Design review of the part built by this model. Coordinates are the model's own, in mm. A direction names the side the tool comes from. Coordinates: 2 decimals unless noted, no trailing zeros. Write each loop counter-clockwise with the first axis right and the second up, starting at its lowest first coordinate (ties: lowest second). Pieces come first, ordered by that corner, then holes.
Q1. Take a section at A-A, the plane x = 11.8. Write out the cut boundary in (y, z), plus the area to 3 significant figures.
Q2. Take a section at B-B, the plane y = 3.5. Write out the cut boundary in (x, z), plus the area to 3 significant figures.
Q3. For pin 1 Ø11 at (x, y) = (-5.5, -1.5) entering from +Z; pin 2 Ø2 at (y, z) = (10.5, -39) entering from +X; pin 3 Ø5 at (x, y) = (-3, 11.5) entering from +Z, all flat-tipped, find the tip position at first contact; note any pin that passes through.
Q4. Take a section at D-D, the plane z = -24. Write out the cut boundary in (x, y).
Q5. For L1, parallel to X at y = 0.25, z = -9.45; L2, parallel to X at y = 5.25, z = 35 (3 decimals); L3, parallel to X at y = 12.25, z = 33.5, list the stretches that pass through material, from the lowest coordinate up.
Q6. For faces 4 (the cylindrical face through (13.11, 0.07, -8.62)), 5 (the flat face through (16.3, 10, 13)), list the 3-axis set-ups (+Z, -Z, +X, -X, +Y, -Y) from which the entire face can be reached by the end or side of a thin tool; tool diameter is ignored.
Q7. Take a section at C-C, the plane z = -9.45. Write out the cut boundary in (x, y).
Q8. The part is to be moulded in two halves that separate along Z. For faces 1 (the flat face through (-17, 10, -38)), 2 (the flat face through (0, 0, 40)), 3 (the flat face through (30, 5, 0)), say which applies: released by +Z, released by -Z, zero draft, split by the parting line, or undercut.
from build123d import *

# Parameters (mm, degrees)
SKETCH1_W           = 60
SKETCH1_H           = 80
BOSS_EXTRUDE1_DEPTH = 5
FILLET1_R           = 10
SKETCH3_R           = 1.55
CUT_EXTRUDE11_DEPTH = 10
BOSS_EXTRUDE2_DEPTH = 10
BOSS_EXTRUDE3_DEPTH = 10


with BuildPart() as part:
    # Sketch1 → Boss-Extrude1 (new, symmetric)
    with BuildSketch(Plane(origin=(0, 0, 0), x_dir=(1, 0, 0), z_dir=(0, 1, 0))):
        Rectangle(SKETCH1_W, SKETCH1_H)
    extrude(amount=BOSS_EXTRUDE1_DEPTH, both=True)

    # Fillet1
    fillet1_edges = [part.edges().sort_by_distance(p)[0] for p in [
        (-30, 0, -40),
        (30, 0, -40),
        (30, 0, 40),
        (-30, 0, 40),
    ]]
    fillet(fillet1_edges, radius=FILLET1_R)

    # Sketch3 → Cut-Extrude11 (cut)
    with BuildSketch(Plane(origin=(0, 5, 0), x_dir=(1, 0, 0), z_dir=(0, 1, 0))):
        with Locations(Location((-11.8, 9.45, 0), (0, 0, 270))):
            Circle(SKETCH3_R)
        with Locations(Location((11.8, 9.45, 0), (0, 0, 270))):
            Circle(SKETCH3_R)
        with Locations(Location((-11.8, -37.55, 0), (0, 0, 270))):
            Circle(SKETCH3_R)
        with Locations(Location((11.8, -37.55, 0), (0, 0, 270))):
            Circle(SKETCH3_R)
    extrude(amount=-CUT_EXTRUDE11_DEPTH, mode=Mode.SUBTRACT)

    # Sketch6 → Boss-Extrude2 (add)
    with BuildSketch(Plane(origin=(0, 5, 0), x_dir=(1, 0, 0), z_dir=(0, 1, 0))):
        with BuildLine():
            Line((30, -30), (30, 30))
            ThreePointArc((30, 30), (27.071067812, 37.071067812), (20, 40))
            Line((20, 40), (14.5, 40))
            Line((14.5, 40), (14.5, 38))
            Line((14.5, 38), (20, 38))
            ThreePointArc((20, 38), (25.656854249, 35.656854249), (28, 30))
            Line((28, 30), (28, -30))
            ThreePointArc((28, -30), (25.652656249, -35.661049137), (19.988130666, -37.999991195))
            Line((19.988130666, -37.999991195), (14.301118682, -38.071478623))
            Line((14.301118682, -38.071478623), (14.285233791, -38.789415009))
            Line((14.285233791, -38.789415009), (12.98648686, -40.088161941))
            Line((12.98648686, -40.088161941), (20, -40))
            ThreePointArc((20, -40), (27.071067812, -37.071067812), (30, -30))
        make_face()
        with BuildLine():
            Line((-30, 30), (-30, -30))
            ThreePointArc((-30, -30), (-27.071067812, -37.071067812), (-20, -40))
            Line((-20, -40), (-13.014230023, -40.088161941))
            Line((-13.014230023, -40.088161941), (-14.314872692, -38.748440589))
            Line((-14.314872692, -38.748440589), (-14.314872692, -38.071588283))
            Line((-14.314872692, -38.071588283), (-19.988083532, -37.999991125))
            ThreePointArc((-19.988083532, -37.999991125), (-25.652639572, -35.661065789), (-28, -30))
            Line((-28, -30), (-28, 30))
            ThreePointArc((-28, 30), (-25.656854249, 35.656854249), (-20, 38))
            Line((-20, 38), (-14.5, 38))
            Line((-14.5, 38), (-14.5, 40))
            Line((-14.5, 40), (-20, 40))
            ThreePointArc((-20, 40), (-27.071067812, 37.071067812), (-30, 30))
        make_face()
    extrude(amount=BOSS_EXTRUDE2_DEPTH)

    # Sketch5 → Boss-Extrude3 (add)
    with BuildSketch(Plane(origin=(0, 5, 0), x_dir=(1, 0, 0), z_dir=(0, 1, 0))):
        Polygon((14.285233791, -38.789415009), (14.3, 10.507634941), (12.98648686, 11.821148081), (-13.014230023, 11.821148081), (-14.31369616, 10.516205754), (-14.314872692, 10.512459037), (-14.314872692, -38.748440589), (-16.314872692, -38.748440589), (-16.314872692, 10.819094366), (-15.842590188, 11.515908447), (-13.84512164, 13.821148081), (13.814913984, 13.821148081), (16.300248159, 11.335813907), (16.300248159, -38.789415009), align=None)
    extrude(amount=BOSS_EXTRUDE3_DEPTH)


solid = part.part
Responses:
1. outline: (-5, -40) - (5, -40) - (5, -13.82) - (15, -13.82) - (15, -11.82) - (5, -11.82) - (5, -11) - (-5, -11) - close; (-5, -7.9) - (5, -7.9) - (5, 36) - (-5, 36) - close; (-5, 39.1) - (5, 39.1) - (5, 40) - (-5, 40) - close
1. area: 758 mm2
2. outline: (-30, -30) arc R10 ccw to (-20, -40) - (20, -40) arc R10 ccw to (30, -30) - (30, 30) arc R10 ccw to (20, 40) - (-20, 40) arc R10 ccw to (-30, 30) - close; hole circle Ø3.1 at (-11.8, -9.45); hole circle Ø3.1 at (-11.8, 37.55); hole circle Ø3.1 at (11.8, -9.45); hole circle Ø3.1 at (11.8, 37.55)
2. area: 4,680 mm2
3. pin 1: stops at z = 40
3. pin 2: stops at x = 26
3. pin 3: stops at z = -11.82
4. outline: (-30, -5) - (30, -5) - (30, 15) - (28, 15) - (28, 5) - (-28, 5) - (-28, 15) - (-30, 15) - close
5. L1: x = -30 to -13.35, -10.25 to 10.25, 13.35 to 30
5. L2: x = -28.66 to -26.245, -16.315 to -14.315, 14.286 to 16.3, 26.245 to 28.66
5. L3: x = -29.37 to -27.19, -16.31 to -14.31, 14.29 to 16.3, 27.19 to 29.37
6. face 4: +Y, -Y
6. face 5: +Y
7. outline: (-30, -5) - (-13.35, -5) - (-13.35, 5) - (-14.31, 5) - (-14.31, 15) - (-16.31, 15) - (-16.31, 5) - (-28, 5) - (-28, 15) - (-30, 15) - close; (-10.25, -5) - (10.25, -5) - (10.25, 5) - (-10.25, 5) - close; (13.35, -5) - (30, -5) - (30, 15) - (28, 15) - (28, 5) - (16.3, 5) - (16.3, 15) - (14.3, 15) - (14.3, 5) - (13.35, 5) - close
8. face 1: undercut
8. face 2: released by +Z
8. face 3: zero draft
